Here's the drawing with two shaded views (mm, measured from the low corner). I have some questions. Give positions to 0.01 mm unless a question says otherwise; leave off trailing zeros. Order: outer loops, then holes, each group sorted by start corner. A loop starts at its lowest first (then second) coordinate and runs counter-clockwise, first axis right, second up. Notation, with made-up numbers: M -15.75,35.5 L 20.25,35.5 A23 ccw 20.25,47.5 Z; hole C 68.5,-25 d2. An arc over 180 degrees is marked long. Use a Markdown table: item, result. Add a question column.
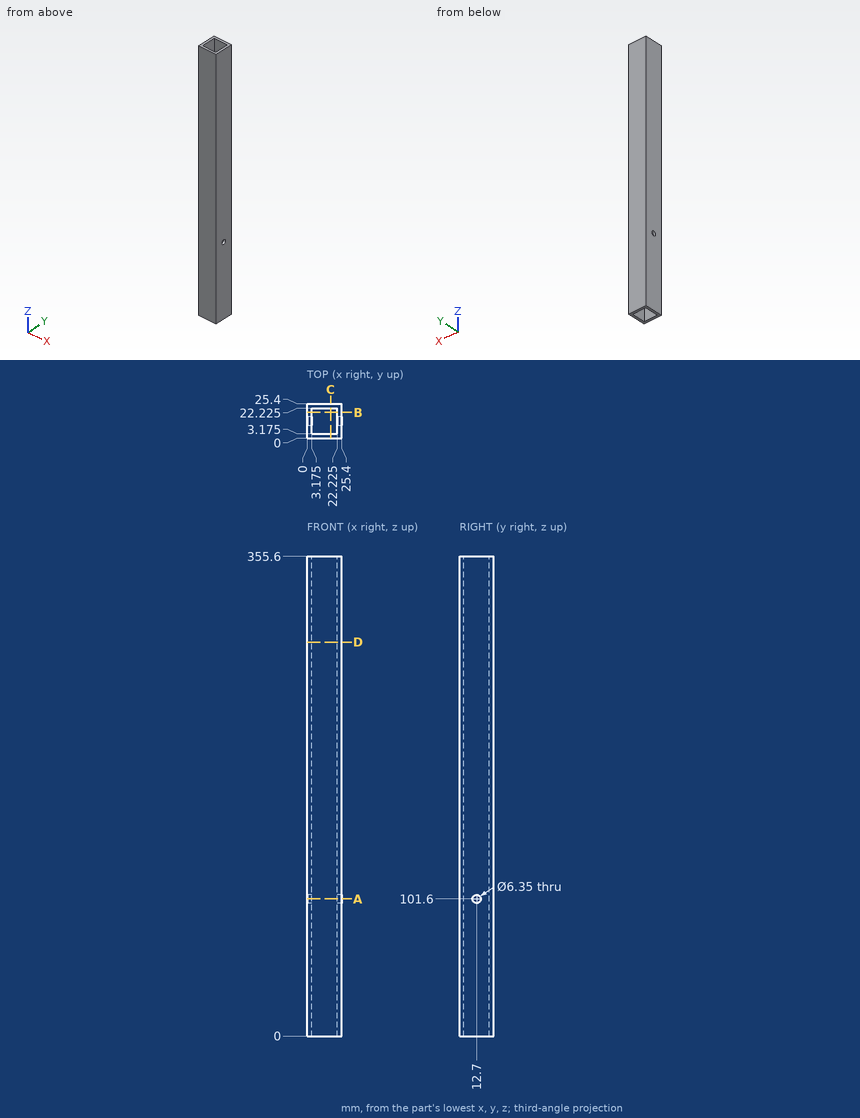
1) Suppose I cut it at D-D on z = 292. Please give me the cut outline in (x, y) (3 decimals), and give its area (3 significant figures).
2) Suppose I cut it at B-B on y = 19.25. Please give me the cut outline in (x, z) (3 decimals), and give its area (3 significant figures).
3) Please list where these lines run through material, in increasing order: line 1 (Y direction, x = 21.75, z = 45) (3 decimals); line 2 (Z direction, x = 1.4, y = 12.7) (3 decimals). Write a range as from..to.
4) For pin 1 (5 mm diameter, centred on y = 12.7, z = 101.6, fed in from -X), with a flat end and sliding along its axis, tell me the tip position at first contact or that it passes through.
5) Suppose I cut it at A-A on z = 101.6. Please give me the cut outline in (x, y) (3 decimals), and give its area (3 significant figures).
Values found:
| question | item | result |
|---|---|---|
| 1 | outline | M 0,0 L 25.4,0 L 25.4,25.4 L 0,25.4 Z; hole M 3.175,3.175 L 22.225,3.175 L 22.225,22.225 L 3.175,22.225 Z |
| 1 | area | 282 mm^2 |
| 2 | outline | M 0,0 L 3.175,0 L 3.175,355.6 L 0,355.6 Z; M 22.225,0 L 25.4,0 L 25.4,355.6 L 22.225,355.6 Z |
| 2 | area | 2,260 mm^2 |
| 3 | line 1 | y = 0..3.175, 22.225..25.4 |
| 3 | line 2 | z = 0..98.425, 104.775..355.6 |
| 4 | pin 1 | passes through |
| 5 | outline | M 0,0 L 25.4,0 L 25.4,9.525 L 22.225,9.525 L 22.225,3.175 L 3.175,3.175 L 3.175,9.525 L 0,9.525 Z; M 0,15.875 L 3.175,15.875 L 3.175,22.225 L 22.225,22.225 L 22.225,15.875 L 25.4,15.875 L 25.4,25.4 L 0,25.4 Z |
| 5 | area | 242 mm^2 |
